from build123d import *

# Parameters (mm, degrees)
EXTRUDE_1_DEPTH     = 10
SKETCH_2_R          = 1.5
CUT_EXTRUDE_1_DEPTH = 2
SKETCH_3_R          = 0.4
EXTRUDE_2_DEPTH     = 3.5


with BuildPart() as part:
    # 草图1 → 凸台-拉伸1 (new body)
    with BuildSketch(Plane(origin=(0, 0, 0), x_dir=(0, 0, -1), z_dir=(1, 0, 0))):
        Polygon((0, 0), (5, 0), (5, 6.798949449), (1.592861235, 14.1), (-1.592861235, 14.1), (-3.462246636, 10.852770352), (-5.2, 10.041823104), (-5.2, 6.798949449), (-3.305827132, 5.708500208), (-3.305827132, 2.534594125), (-5.2, 1.506142854), (-5.2, 0), align=None)
    extrude(amount=EXTRUDE_1_DEPTH)

    # 草图2 → 切除-拉伸1 (cut)
    with BuildSketch(Plane(origin=(0, 14.1, 0), x_dir=(1, 0, 0), z_dir=(0, 1, 0))):
        with Locations(Location((2.54, 0, 0), (0, 0, 270))):
            Circle(SKETCH_2_R)
        with Locations(Location((7.54, 0, 0), (0, 0, 270))):
            Circle(SKETCH_2_R)
    extrude(amount=-CUT_EXTRUDE_1_DEPTH, mode=Mode.SUBTRACT)

    # 草图3 → 凸台-拉伸2 (add)
    with BuildSketch(Plane.XZ):
        with Locations(Location((2.5, 0, 0), (0, 0, 90))):
            Circle(SKETCH_3_R)
        with Locations(Location((7.5, 0, 0), (0, 0, 90))):
            Circle(SKETCH_3_R)
    extrude(amount=EXTRUDE_2_DEPTH)


solid = part.part
Here's how the part is built. I have some questions about the finished solid (model axes, mm). A direction names the side the tool comes from. Coordinates: 2 decimals unless noted, no trailing zeros. Loops run counter-clockwise (first coordinate to the right, second up) from the corner with the lowest first, then second, coordinate; pieces in that order, holes last.
1. If we mould it in two halves opening along X, with no side actions, what happens to faces 1 (the flat face through (0, 7, 0)), 2 (the cylindrical face through (9.027, 13.114, -0.195)), 3 (the flat face through (10, 7, 0)), 4 (the flat face through (5, 8, 5.2))? For each: pulls with the +X half, pulls with the -X half, needs draft (parallel to the pull), parting line crosses it, or undercut.
2. For P1, Ø2.5, axis at x = 2.54, z = 0, coming from the +Y side; P2, Ø4, axis at x = 8.5, y = 12, coming from the -Z side; P3, Ø3.5, axis at x = 6, y = 4.5, coming from the +Z side, each with a flat end and sliding along its axis, tell me the tip position at first contact or that it passes through.
3. Imagine slicing it at C-C, the plane y = 12.75. Please give me the cut outline in (x, z).
4. Imagine slicing it at A-A, the plane x = 5. Please give me the cut outline in (y, z), and give its area (3 significant figures).
5. For faces 5 (the flat face through (4.93, 6.261, 4.266)), 6 (the cylindrical face through (7.103, -1.726, -0.052)), 7 (the flat face through (3, 12.1, 0)), 8 (the flat face through (4.93, 12.499, 2.514)), 9 (the flat face through (5, 14.1, 0)), which set-ups out of +Z, -Z, +X, -X, +Y, -Y let a thin tool reach every point of the face, with its end or its side?
6. I need wall thicknesses on L1, parallel to X at y = 13.2, z = 0; L2, parallel to Z at x = 8, y = 3.75; L3, parallel to Y at x = 2.25, z = 4. Which ranges of each line are inside material? Lowest first, please.
7. Imagine slicing it at B-B, the plane z = 0. Please give me the cut outline in (x, y).
8. Imagine slicing it at D-D, the plane x = 1.5. Please give me the cut outline in (y, z), and give its area (3 significant figures).
Taken from the geometry:
1. face 1: pulls with the -X half
1. face 2: undercut
1. face 3: pulls with the +X half
1. face 4: needs draft
2. P1: stops at y = 12.1
2. P2: stops at z = -3.51
2. P3: stops at z = 4.25
3. outline: (0, -2.22) - (10, -2.22) - (10, 2.37) - (0, 2.37) - close; hole circle Ø3 at (2.54, 0); hole circle Ø3 at (7.54, 0)
4. outline: (0, -5) - (6.8, -5) - (14.1, -1.59) - (14.1, 1.59) - (10.85, 3.46) - (10.04, 5.2) - (6.8, 5.2) - (5.71, 3.31) - (2.53, 3.31) - (1.51, 5.2) - (0, 5.2) - close
4. area: 114 mm2
5. face 5: +Z, +X, -X
5. face 6: -Y
5. face 7: +Y
5. face 8: +Z, +X, -X, +Y
5. face 9: +Z, -Z, +X, -X, +Y
6. L1: x = 0 to 1.04, 4.04 to 6.04, 9.04 to 10
6. L2: z = -5 to 3.31
6. L3: y = 0 to 2.16, 6.11 to 10.6
7. outline: (0, 0) - (2.1, 0) - (2.1, -3.5) - (2.9, -3.5) - (2.9, 0) - (7.1, 0) - (7.1, -3.5) - (7.9, -3.5) - (7.9, 0) - (10, 0) - (10, 14.1) - (9.04, 14.1) - (9.04, 12.1) - (6.04, 12.1) - (6.04, 14.1) - (4.04, 14.1) - (4.04, 12.1) - (1.04, 12.1) - (1.04, 14.1) - (0, 14.1) - close
8. outline: (0, -5) - (6.8, -5) - (14.1, -1.59) - (14.1, -1.08) - (12.1, -1.08) - (12.1, 1.08) - (14.1, 1.08) - (14.1, 1.59) - (10.85, 3.46) - (10.04, 5.2) - (6.8, 5.2) - (5.71, 3.31) - (2.53, 3.31) - (1.51, 5.2) - (0, 5.2) - close
8. area: 110 mm2
